Design review of the part shown in the three views and the two pictorial views. Dimensions are in mm from the part's minimum x, y and z. Coordinates: 2 decimals unless noted, no trailing zeros. Loops run counter-clockwise (first coordinate to the right, second up) from the corner with the lowest first, then second, coordinate; pieces in that order, holes last. Notation, with made-up numbers: M 8,42 L 30,42 A16 ccw 30,62 Z; hole C 5.5,73 d11. An arc over 180 degrees is marked long. Put each result on its own line as item: value. Start each with the question number.
(1) Clearance check with flat-ended pins moving along their axes: pin 1 (3 mm diameter, centred on y = 2.5, z = 3.5, fed in from +X); pin 2 (1.7 mm diameter, centred on y = 4, z = 1.5, fed in from -X); pin 3 (3 mm diameter, centred on x = 144, z = 2.5, fed in from -Y); pin 4 (4.5 mm diameter, centred on x = 144.5, y = 57.4, fed in from -Z). State where each tip first meets the part, or that it passes through.
(2) Take a section at B-B, the plane y = 36.4. Give the boundary of the cut face in (x, z), then the cut area to 3 significant figures.
(3) Take a section at C-C, the plane z = 2.05. Give the boundary of the cut face in (x, y).
(4) Take a section at A-A, the plane x = 144.5. Give the boundary of the cut face in (y, z), then the cut area to 3 significant figures.
(5) For probe 1 along X at (y, z) = (36, 1.95); probe 2 along X at (y, z) = (57.4, 1.95); probe 3 along Y at (x, z) = (144.5, 4.25), list the stretches that pass through material, from the lowest coordinate up. Write a range as [from, to].
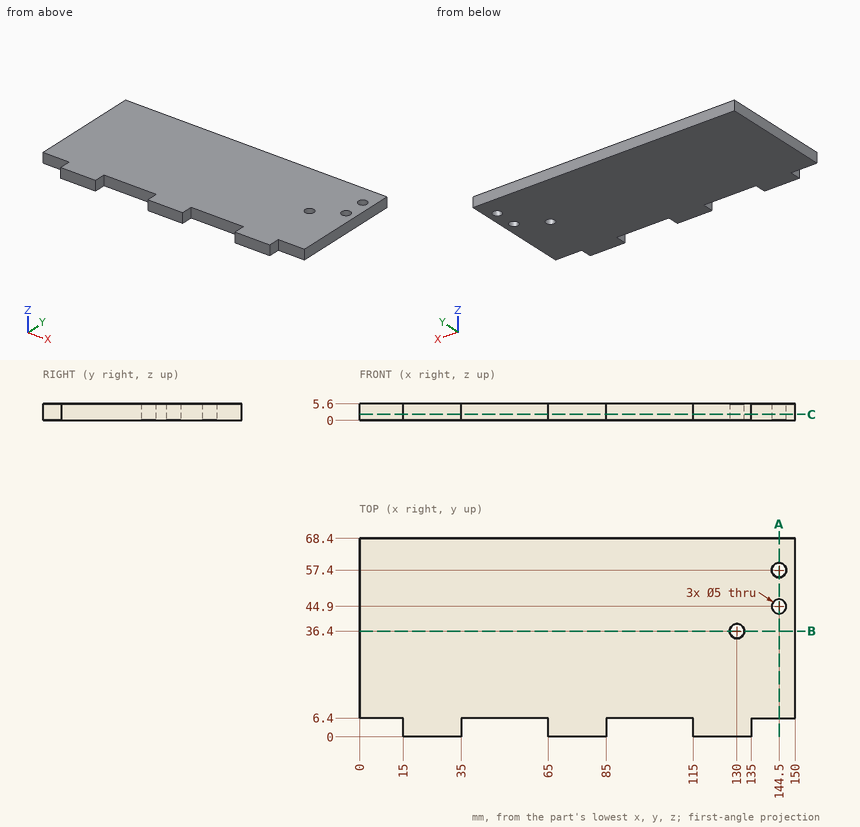
Computed values:
1. pin 1: stops at x = 135
1. pin 2: stops at x = 15
1. pin 3: stops at y = 6.4
1. pin 4: passes through
2. outline: M 0,0 L 127.5,0 L 127.5,5.6 L 0,5.6 Z; M 132.5,0 L 150,0 L 150,5.6 L 132.5,5.6 Z
2. area: 812 mm^2
3. outline: M 0,6.4 L 15,6.4 L 15,0 L 35,0 L 35,6.4 L 65,6.4 L 65,0 L 85,0 L 85,6.4 L 115,6.4 L 115,0 L 135,0 L 135,6.4 L 150,6.4 L 150,68.4 L 0,68.4 Z; hole C 130,36.4 d5; hole C 144.5,44.9 d5; hole C 144.5,57.4 d5
4. outline: M 6.4,0 L 42.4,0 L 42.4,5.6 L 6.4,5.6 Z; M 47.4,0 L 54.9,0 L 54.9,5.6 L 47.4,5.6 Z; M 59.9,0 L 68.4,0 L 68.4,5.6 L 59.9,5.6 Z
4. area: 291 mm^2
5. probe 1: x = [0, 127.53], [132.47, 150]
5. probe 2: x = [0, 142], [147, 150]
5. probe 3: y = [6.4, 42.4], [47.4, 54.9], [59.9, 68.4]
